from build123d import *

# Parameters (mm, degrees)
SKETCH1_R                = 5
BOSS_EXTRUDE1_DEPTH      = 4
BOSS_EXTRUDE2_START      = 4
SKETCH2_R                = 5
BOSS_EXTRUDE2_DEPTH      = 4
BOSS_EXTRUDE5_DEPTH      = 15
BOSS_EXTRUDE5_DEPTH_BACK = 7
SKETCH5_R                = 4
CUT_EXTRUDE1_DEPTH       = 17.807438829
CUT_EXTRUDE1_DEPTH_BACK  = 17.807438829
SKETCH9_R                = 1


with BuildPart() as part:
    # Sketch1 → Boss-Extrude1 (new body)
    with BuildSketch(Plane.XY):
        with Locations((0, 0.7)):
            Circle(SKETCH1_R)
    extrude(amount=BOSS_EXTRUDE1_DEPTH)

    # Sketch2 → Boss-Extrude2 (add)
    with BuildSketch(Plane.XY.offset(BOSS_EXTRUDE2_START)):
        with Locations(Location((0, -0.7, 0), (0, 0, 171.952153753))):
            Circle(SKETCH2_R)
    extrude(amount=BOSS_EXTRUDE2_DEPTH)

    # Sketch5 → Boss-Extrude5 (add, two sides: drawn at the far end of the back side and taken through both)
    with BuildSketch(Plane.XY.offset(-BOSS_EXTRUDE5_DEPTH_BACK)):
        Circle(SKETCH5_R)
    extrude(amount=BOSS_EXTRUDE5_DEPTH + BOSS_EXTRUDE5_DEPTH_BACK)

    # Sketch9 → Cut-Extrude1 (cut, two sides: drawn at the far end of the back side and taken through both)
    with BuildSketch(Plane.XY.offset(-CUT_EXTRUDE1_DEPTH_BACK)):
        with BuildLine():
            ThreePointArc((0, 3.3), (-1, 2.3), (0, 1.3))
            Line((0, 1.3), (0, 3.3))
        make_face()
        with BuildLine():
            Line((0, 3.3), (0, 1.3))
            ThreePointArc((0, 1.3), (0.707106781, 1.592893219), (1, 2.3))
            ThreePointArc((1, 2.3), (0.707106781, 3.007106781), (0, 3.3))
        make_face()
        with Locations((-1.991858429, -1.15)):
            Circle(SKETCH9_R)
        with Locations((1.991858429, -1.15)):
            Circle(SKETCH9_R)
    extrude(amount=CUT_EXTRUDE1_DEPTH + CUT_EXTRUDE1_DEPTH_BACK, mode=Mode.SUBTRACT)


solid = part.part
Work out the finished part from the listing and answer in its coordinate system (mm). A direction names the side the tool comes from. Coordinates: 2 decimals unless noted, no trailing zeros. Write each loop counter-clockwise with the first axis right and the second up, starting at its lowest first coordinate (ties: lowest second). Pieces come first, ordered by that corner, then holes.
1. For faces 1 (the flat face through (0, 5, 4)), 2 (the flat face through (-2, -4, 8)), 3 (the flat face through (0, -5, 4)), 4 (the flat face through (0, 4.4, 0)), determine the directions among +Z, -Z, +X, -X, +Y, -Y from which every point of the face is accessible in a straight line to the end or side of a thin tool.
Results list:
face 1: +Z, +Y
face 2: +Z
face 3: -Z, -Y
face 4: -Z
2. The part is cut by section B-B, the plane x = -0.25. Write down the section's boundary in (y, z).
Results list:
outline: (-5.69, 4) - (-4.29, 4) - (-4.29, 0) - (-3.99, 0) - (-3.99, -7) - (1.33, -7) - (1.33, 15) - (-3.99, 15) - (-3.99, 8) - (-5.69, 8) - close; (3.27, -7) - (3.99, -7) - (3.99, 0) - (5.69, 0) - (5.69, 4) - (4.29, 4) - (4.29, 8) - (3.99, 8) - (3.99, 15) - (3.27, 15) - close
3. Consider line 1 along X through (y, z) = (-1.15, 2); line 2 along X through (y, z) = (-1.15, 6.5); line 3 along Y through (x, z) = (0.75, 7.5). Determine where each line is inside the solid, lowest interval first.
Results list:
line 1: x = -4.65 to -2.99, -0.99 to 0.99, 2.99 to 4.65
line 2: x = -4.98 to -2.99, -0.99 to 0.99, 2.99 to 4.98
line 3: y = -5.64 to 1.64, 2.96 to 4.24
4. The part is cut by section D-D, the plane x = -4.25. Write down the section's boundary in (y, z).
Results list:
outline: (-3.33, 4) - (-1.93, 4) - (-1.93, 0) - (3.33, 0) - (3.33, 4) - (1.93, 4) - (1.93, 8) - (-3.33, 8) - close
5. Flat-ended cylindrical pins translate along their axes: pin 1 (1 mm diameter, centred on y = -3, z = 13, fed in from -X); pin 2 (1.8 mm diameter, centred on x = -1.99, y = -1.15, fed in from +Z); pin 3 (2 mm diameter, centred on x = -3.5, z = 8.5, fed in from +Y); pin 4 (5 mm diameter, centred on y = 3.5, z = 12.5, fed in from +X). Find the tip coordinate at first contact, or state that the pin passes through.
Results list:
pin 1: stops at x = -3.12
pin 2: passes through
pin 3: stops at y = 3.55
pin 4: stops at x = 3.87
6. The part is cut by section A-A, the plane y = -1.5. Write down the section's boundary in (x, z), and give its area (3 significant figures).
Results list:
outline: (-4.94, 4) - (-4.49, 4) - (-4.49, 0) - (-3.71, 0) - (-3.71, -7) - (-2.93, -7) - (-2.93, 15) - (-3.71, 15) - (-3.71, 8) - (-4.94, 8) - close; (-1.06, -7) - (1.06, -7) - (1.06, 15) - (-1.06, 15) - close; (2.93, -7) - (3.71, -7) - (3.71, 0) - (4.49, 0) - (4.49, 4) - (4.94, 4) - (4.94, 8) - (3.71, 8) - (3.71, 15) - (2.93, 15) - close
area: 96.8 mm2
7. The part is cut by section C-C, the plane z = -5. Write down the section's boundary in (x, y), and give its area (3 significant figures).
Results list:
outline: circle Ø8 at (0, 0); hole circle Ø2 at (-1.99, -1.15); hole circle Ø2 at (0, 2.3); hole circle Ø2 at (1.99, -1.15)
area: 40.8 mm2
8. For a pull along Y with two mould halves and no side action, classify faces 5 (the flat face through (0, 0, -7)), 6 (the cylindrical face through (-0.867, -3.905, -3.549)), 7 (the cylindrical face through (-2.209, -2.126, 3.846)) as +Y half, -Y half, draft (parallel to the pull), parting line (faces both ways), or undercut.
Results list:
face 5: draft
face 6: parting line
face 7: undercut
